Read the model definition and answer for the solid it produces. Units are mm, in the model's axes. A direction names the side the tool comes from. Round coordinates to 2 decimals unless told otherwise and drop trailing zeros. Write each loop counter-clockwise with the first axis right and the second up, starting at its lowest first coordinate (ties: lowest second). Pieces come first, ordered by that corner, then holes.
from build123d import *

# Parameters (mm, degrees)
PAD017_DEPTH    = 10
POCKET021_DEPTH = 12.5
SKETCH043_R     = 3.4
POCKET022_DEPTH = 9.5
SKETCH042_R     = 4.75
POCKET023_DEPTH = 6
SKETCH044_R     = 3.25
POCKET024_DEPTH = 9.5
CHAMFER003_SIZE = 0.5
SKETCH045_W     = 10
SKETCH045_H     = 3.416477
POCKET025_DEPTH = 5


with BuildPart() as part:
    # Sketch040 → Pad017 (new body, symmetric)
    with BuildSketch(Plane.YZ):
        Polygon((-6.020616, 5), (-6.020616, 0), (6.020616, 0), (11.979384, 5), (11.979384, 18), (-6.020616, 18), align=None)
    extrude(amount=PAD017_DEPTH, both=True)

    # Sketch041 → Pocket021 (cut, symmetric)
    with BuildSketch(Plane.XZ):
        Polygon((-2.85926, 0), (-10, 5), (-10, 0), align=None)
    extrude(amount=POCKET021_DEPTH, both=True, mode=Mode.SUBTRACT)

    # Sketch043 (on Face7 of Pocket021) → Pocket022 (cut)
    with BuildSketch(Plane.ZX.offset(11.979384)):
        with Locations((11.617009, -4.472668)):
            Circle(SKETCH043_R)
    extrude(amount=-POCKET022_DEPTH, mode=Mode.SUBTRACT)

    # Sketch042 (on Face5 of Pocket021) → Pocket023 (cut)
    with BuildSketch(Plane(origin=(0, -6.020616, 0), x_dir=(0, 0, -1), z_dir=(0, -1, 0))):
        with Locations((-10.693305, -2.090455)):
            Circle(SKETCH042_R)
    extrude(amount=-POCKET023_DEPTH, mode=Mode.SUBTRACT)

    # Sketch044 (on Face4 of Pocket023) → Pocket024 (cut)
    with BuildSketch(Plane.YZ.offset(10)):
        with Locations((4.93403, 6.679259)):
            Circle(SKETCH044_R)
    extrude(amount=-POCKET024_DEPTH, mode=Mode.SUBTRACT)

    # Chamfer003
    chamfer003_edges = [part.edges().sort_by_distance(p)[0] for p in [
        (-4.472668, 11.979384, 8.217009),
        (10, 1.68403, 6.679259),
        (-2.090455, -6.020616, 15.443305),
    ]]
    chamfer(chamfer003_edges, length=CHAMFER003_SIZE)

    # Sketch045 (on Face1 of Chamfer003) → Pocket025 (cut)
    with BuildSketch(Plane.YZ.offset(10)):
        with Locations((2.746655, 14.302369)):
            Rectangle(SKETCH045_W, SKETCH045_H)
    extrude(amount=-POCKET025_DEPTH, mode=Mode.SUBTRACT)


solid = part.part
Q1. Section C-C (z = 2) is taken. Determine the outline of the cut face in (x, y), then the cut area to 3 significant figures.
Verdict:
outline: (-5.72, -6.02) - (10, -6.02) - (10, 8.4) - (-5.72, 8.4) - close
area: 227 mm2
Q2. Section A-A (y = 10.25) is taken. Determine the outline of the cut face in (x, z), then the cut area to 3 significant figures.
Verdict:
outline: (-10, 5) - (-7.93, 3.55) - (10, 3.55) - (10, 18) - (-10, 18) - close; hole circle Ø6.8 at (-4.47, 11.62)
area: 251 mm2
Q3. Section B-B (x = 5.75) is taken. Determine the outline of the cut face in (y, z), then the cut area to 3 significant figures.
Verdict:
outline: (-6.02, 0) - (6.02, 0) - (11.98, 5) - (11.98, 18) - (-6.02, 18) - close; hole (-2.25, 12.59) - (7.75, 12.59) - (7.75, 16.01) - (-2.25, 16.01) - close; hole circle Ø6.5 at (4.93, 6.68)
area: 242 mm2
Q4. Determine the mould class of faces 5 (the flat face through (0.5, 5, 7)), 6 (the flat face through (-6.38, 0.853, 2.465)), 7 (the flat face through (2.4, 9, 2.5)) for opening direction Y: pulls with the +Y half, pulls with the -Y half, needs draft (parallel to the pull), parting line crosses it, or undercut.
Verdict:
face 5: undercut
face 6: needs draft
face 7: pulls with the +Y half
Q5. Straight lines are drawn through the part: probe 1 along Z at (x, y) = (9, 1); probe 2 along Z at (x, y) = (6.5, 7); probe 3 along Y at (x, z) = (6.75, 7). For each, find the intervals that lie inside material, in ascending order.
Verdict:
probe 1: z = 0 to 12.59, 16.01 to 18
probe 2: z = 0.82 to 4.17, 9.19 to 12.59, 16.01 to 18
probe 3: y = -6.02 to 1.7, 8.17 to 11.98
Q6. Flat-ended cylindrical pins translate along their axes: pin 1 Ø5 at (x, z) = (-2.5, 9) entering from -Y; pin 2 Ø8 at (x, y) = (0, 4) entering from -Z; pin 3 Ø1.7 at (y, z) = (4.5, 13.5) entering from +X; pin 4 Ø4 at (x, z) = (-4.47, 11.62) entering from +Y. Find the tip coordinate at first contact, or state that the pin passes through.
Verdict:
pin 1: stops at y = -0.02
pin 2: stops at z = 0
pin 3: stops at x = 5
pin 4: stops at y = 2.48
Q7. Which of the six approach directions +Z, -Z, +X, -X, +Y, -Y give full straight-line access (tool end or side, diameter ignored) to faces 1 (the flat face through (0, 3, 18)), 2 (the flat face through (5, 3, 14)), 3 (the cylindrical face through (-1.88, -2.81, 15.44)), 4 (the flat face through (-4, 2.479, 12))?
Verdict:
face 1: +Z, +X, -X, +Y, -Y
face 2: +X
face 3: -Y
face 4: +Y
Q8. Section D-D (y = -1.25) is taken. Determine the outline of the cut face in (x, z).
Verdict:
outline: (-10, 5) - (-2.86, 0) - (10, 0) - (10, 12.59) - (5, 12.59) - (5, 16.01) - (10, 16.01) - (10, 18) - (-10, 18) - close; hole circle Ø9.5 at (-2.09, 10.69)
